Build history of the part. All positions in model axes, mm. Coordinates: 2 decimals unless noted, no trailing zeros. Write each loop counter-clockwise with the first axis right and the second up, starting at its lowest first coordinate (ties: lowest second). Pieces come first, ordered by that corner, then holes.
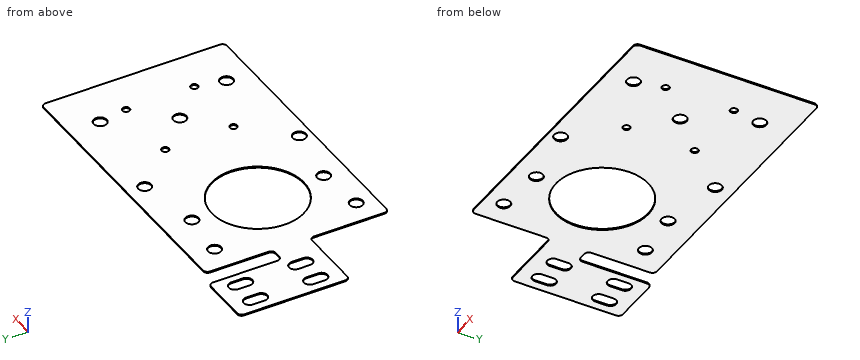
Autodesk Inventor part; units mm, degrees
ref_plane "YZ Plane" through (0, 0, 0) normal (1, 0, 0) x (0, 1, 0)
ref_plane "XZ Plane" through (0, 0, 0) normal (0, 1, 0) x (-1, 0, 0)
ref_plane "XY Plane" through (0, 0, 0) normal (0, 0, 1) x (1, 0, 0)
sketch "Boceto1" plane through (0, 0, 0) normal (0, 0, 1) x (1, 0, 0)
  line L0 (-122.755, 65.145) -> (122.755, -65.145) construction
  line L1 (122.755, 65.145) -> (-122.755, -65.145) construction
  line L2 (-122.755, 65.145) -> (-85.295, 65.145)
  line L3 (-122.755, 65.145) -> (-122.755, -10.585)
  line L4 (-85.295, 65.145) -> (-85.295, 14.655)
  line L5 (-85.295, 14.655) -> (-74.705, 14.655)
  line L6 (-74.705, 14.655) -> (-74.705, 61.075)
  line L7 (-74.705, 61.075) -> (122.755, 61.075)
  line L8 (-122.755, -10.585) -> (-74.705, -10.585)
  line L9 (-74.705, -10.585) -> (-74.705, -65.145)
  line L10 (-74.705, -65.145) -> (122.755, -65.145)
  line L11 (122.755, 61.075) -> (122.755, -65.145)
  line L12 (122.755, 61.075) -> (122.755, -4.07)
  circle A0 centre (93.325, -27.57) radius 2.5
  circle A1 centre (93.325, 19.43) radius 2.5
  circle A2 centre (46.325, 19.43) radius 2.5
  circle A3 centre (46.325, -27.57) radius 2.5
  line L13 (122.755, 61.075) -> (122.755, -4.07)
  line L14 (122.755, 61.075) -> (122.755, -4.07)
  line L15 (122.755, 61.075) -> (122.755, -4.07)
  circle A4 centre (69.825, -4.07) radius 4.5
  circle A5 centre (90.185, 39.09) radius 4.5
  circle A6 centre (88.9646, -47.2127) radius 4.5
  circle A7 centre (19.745, 48.86) radius 4.5
  circle A8 centre (-56.385, 44.38) radius 4.5
  circle A9 centre (-57.6054, -52.5027) radius 4.5
  circle A10 centre (18.5246, -56.9827) radius 4.5
  circle A11 centre (-23.815, 41.325) radius 4.5
  circle A12 centre (-23.815, -49.465) radius 4.5
  circle A13 centre (-23.815, -4.07) radius 31.755
  line L16 (-116.6465, 10.975) -> (-116.6465, 2.875)
  line L17 (-108.5035, 2.875) -> (-108.5035, 10.975)
  arc A14 (-108.5035, 10.975) -> (-116.6465, 10.975) centre (-112.575, 10.975) ccw
  arc A15 (-116.6465, 2.875) -> (-108.5035, 2.875) centre (-112.575, 2.875) ccw
  line L18 (-98.7365, 10.975) -> (-98.7365, 2.875)
  line L19 (-90.5935, 2.875) -> (-90.5935, 10.975)
  arc A16 (-90.5935, 10.975) -> (-98.7365, 10.975) centre (-94.665, 10.975) ccw
  arc A17 (-98.7365, 2.875) -> (-90.5935, 2.875) centre (-94.665, 2.875) ccw
  line L20 (-116.6465, 52.505) -> (-116.6465, 44.405)
  line L21 (-108.5035, 44.405) -> (-108.5035, 52.505)
  line L22 (-90.5935, 52.505) -> (-90.5935, 44.405)
  line L23 (-98.7365, 44.405) -> (-98.7365, 52.505)
  arc A18 (-108.5035, 52.505) -> (-116.6465, 52.505) centre (-112.575, 52.505) ccw
  arc A19 (-116.6465, 44.405) -> (-108.5035, 44.405) centre (-112.575, 44.405) ccw
  arc A20 (-98.7365, 44.405) -> (-90.5935, 44.405) centre (-94.665, 44.405) ccw
  arc A21 (-90.5935, 52.505) -> (-98.7365, 52.505) centre (-94.665, 52.505) ccw
  point P0 (0, 0)
  point P1 (-112.575, 65.145)
  point P2 (-94.665, 65.145)
  dimension "d0" = 245.51
  dimension "d1" = 130.29
  dimension "d2" = 37.46
  dimension "d3" = 75.73
  dimension "d18" = 5
  dimension "d19" = 5
  dimension "d20" = 5
  dimension "d21" = 5
  dimension "d27" = 9
  dimension "d28" = 9
  dimension "d29" = 9
  dimension "d34" = 9
  dimension "d35" = 9
  dimension "d40" = 9
  dimension "d41" = 9
  dimension "d45" = 9
  dimension "d46" = 9
  dimension "d47" = 63.51
extrude "Extrusión2" add sketch "Boceto1" along normal mid plane 0.8
fillet "Empalme2" radius 3 10 edges at (-85.295, 14.655, 0) (-74.705, 14.655, 0) (-85.295, 65.145, 0) (-122.755, 65.145, 0) (-74.705, 61.075, 0) (122.755, 61.075, 0) (122.755, -65.145, 0) (-74.705, -65.145, 0) (-74.705, -10.585, 0) (-122.755, -10.585, 0)
properties part number "piezaaa"
1. Saw through at C-C on y = -20. List the corners of the cut face in (x, z) (3 decimals), plus the area to 3 significant figures.
Computed values:
outline: (-74.705, -0.4) - (-51.285, -0.4) - (-51.285, 0.4) - (-74.705, 0.4) - close; (3.655, -0.4) - (122.755, -0.4) - (122.755, 0.4) - (3.655, 0.4) - close
area: 114 mm2
2. Probe line 1 along Y through (x, z) = (-25, -0.05) (3 decimals); line 2 along Y through (x, z) = (87.5, -0.1) (3 decimals); line 3 along Y through (x, z) = (92, -0.2) (3 decimals). List the from-to ranges inside material, lowest first.
Computed values:
line 1: y = -65.145 to -53.806, -45.124 to -35.803, 27.663 to 36.984, 45.666 to 61.075
line 2: y = -65.145 to -51.468, -42.958 to 35.479, 42.701 to 61.075
line 3: y = -65.145 to -50.535, -43.891 to -29.69, -25.45 to 17.31, 21.55 to 34.972, 43.208 to 61.075
3. Saw through at A-A on y = -4.07. List the corners of the cut face in (x, z) (3 decimals), plus the area to 3 significant figures.
Computed values:
outline: (-122.755, -0.4) - (-55.57, -0.4) - (-55.57, 0.4) - (-122.755, 0.4) - close; (7.94, -0.4) - (65.325, -0.4) - (65.325, 0.4) - (7.94, 0.4) - close; (74.325, -0.4) - (122.755, -0.4) - (122.755, 0.4) - (74.325, 0.4) - close
area: 138 mm2
4. Saw through at B-B on x = -15. List the corners of the cut face in (y, z) (3 decimals).
Computed values:
outline: (-65.145, -0.4) - (-34.577, -0.4) - (-34.577, 0.4) - (-65.145, 0.4) - close; (26.437, -0.4) - (61.075, -0.4) - (61.075, 0.4) - (26.437, 0.4) - close
5. Saw through at D-D on x = 33.5. List the corners of the cut face in (y, z) (3 decimals).
Computed values:
outline: (-65.145, -0.4) - (61.075, -0.4) - (61.075, 0.4) - (-65.145, 0.4) - close
6. Flat gauge pins, fed straight in: pin 1 (14.5 mm diameter, centred on x = -57.61, y = -52.5, fed in from +Z); pin 2 (8 mm diameter, centred on x = 19.745, y = 48.86, fed in from +Z). Where does each tip first touch, or does it go through?
Computed values:
pin 1: stops at z = 0.4
pin 2: passes through
